Autodesk Inventor part; units mm, degrees
ref_plane "YZ Plane" through (0, 0, 0) normal (1, 0, 0) x (0, 1, 0)
ref_plane "XZ Plane" through (0, 0, 0) normal (0, 1, 0) x (-1, 0, 0)
ref_plane "XY Plane" through (0, 0, 0) normal (0, 0, 1) x (1, 0, 0)
sketch "Sketch1" plane through (0, 0, 0) normal (0, 0, 1) x (1, 0, 0)
  line L0 (-150, -75) -> (150, -75) construction
  line L1 (150, -75) -> (150, 75) construction
  line L2 (150, 75) -> (-150, 75) construction
  line L3 (-150, 75) -> (-150, -75) construction
  line L4 (-150, -75) -> (150, 75) construction
  line L5 (150, -75) -> (-150, 75) construction
  line L6 (147.5, -72.5) -> (-147.5, -72.5) construction
  line L7 (-147.5, -72.5) -> (-147.5, 72.5) construction
  line L8 (-147.5, 72.5) -> (147.5, 72.5) construction
  line L9 (147.5, 72.5) -> (147.5, -72.5) construction
  line L10 (147.5, -72.5) -> (-147.5, 72.5) construction
  line L11 (-147.5, -72.5) -> (147.5, 72.5) construction
  line L12 (-150, 75) -> (-146, 75) construction
  line L13 (-146, 75) -> (-146, 71) construction
  line L14 (-146, 71) -> (-150, 71) construction
  line L15 (-150, 71) -> (-150, 75) construction
  arc A0 (-146, 75) -> (-150, 71) centre (-146, 71) ccw
  line L16 (-150, -75) -> (-146, -75) construction
  line L17 (-146, -75) -> (-146, -71) construction
  line L18 (-146, -71) -> (-150, -71) construction
  line L19 (-150, -71) -> (-150, -75) construction
  line L20 (150, -75) -> (146, -75) construction
  line L21 (146, -75) -> (146, -71) construction
  line L22 (146, -71) -> (150, -71) construction
  line L23 (150, -71) -> (150, -75) construction
  line L24 (150, 75) -> (146, 75) construction
  line L25 (146, 75) -> (146, 71) construction
  line L26 (146, 71) -> (150, 71) construction
  line L27 (150, 71) -> (150, 75) construction
  line L28 (-146, 75) -> (146, 75)
  arc A1 (150, 71) -> (146, 75) centre (146, 71) ccw
  line L29 (150, 71) -> (150, -71)
  arc A2 (146, -75) -> (150, -71) centre (146, -71) ccw
  line L30 (146, -75) -> (-146, -75)
  arc A3 (-150, -71) -> (-146, -75) centre (-146, -71) ccw
  line L31 (-150, -71) -> (-150, 71)
  circle A4 centre (-146, 71) radius 2.5
  circle A5 centre (-146, -71) radius 2.5
  circle A6 centre (146, -71) radius 2.5
  circle A7 centre (146, 71) radius 2.5
  line L32 (-146, 71) -> (-142, 71) construction
  line L33 (-142, 71) -> (-142, 67) construction
  line L34 (-142, 67) -> (-146, 67) construction
  line L35 (-146, 67) -> (-146, 71) construction
  line L36 (-146, -71) -> (-142, -71) construction
  line L37 (-142, -71) -> (-142, -67) construction
  line L38 (-142, -67) -> (-146, -67) construction
  line L39 (-146, -67) -> (-146, -71) construction
  line L40 (146, -71) -> (142, -71) construction
  line L41 (142, -71) -> (142, -67) construction
  line L42 (142, -67) -> (146, -67) construction
  line L43 (146, -67) -> (146, -71) construction
  line L44 (146, 71) -> (142, 71) construction
  line L45 (142, 71) -> (142, 67) construction
  line L46 (142, 67) -> (146, 67) construction
  line L47 (146, 67) -> (146, 71) construction
  arc A8 (-146, 67) -> (-142, 71) centre (-146, 71) ccw
  arc A9 (-142, -71) -> (-146, -67) centre (-146, -71) ccw
  arc A10 (146, -67) -> (142, -71) centre (146, -71) ccw
  arc A11 (142, 71) -> (146, 67) centre (146, 71) ccw
  line L48 (-142, 71) -> (-140.5, 71) construction
  line L49 (-140.5, 71) -> (-140.5, 72.5) construction
  line L50 (-140.5, 72.5) -> (-142, 72.5) construction
  line L51 (-142, 72.5) -> (-142, 71) construction
  line L52 (-146, 67) -> (-147.5, 67) construction
  line L53 (-147.5, 67) -> (-147.5, 65.5) construction
  line L54 (-147.5, 65.5) -> (-146, 65.5) construction
  line L55 (-146, 65.5) -> (-146, 67) construction
  line L56 (142, 71) -> (140.5, 71) construction
  line L57 (140.5, 71) -> (140.5, 72.5) construction
  line L58 (140.5, 72.5) -> (142, 72.5) construction
  line L59 (142, 72.5) -> (142, 71) construction
  line L60 (146, 67) -> (147.5, 67) construction
  line L61 (147.5, 67) -> (147.5, 65.5) construction
  line L62 (147.5, 65.5) -> (146, 65.5) construction
  line L63 (146, 65.5) -> (146, 67) construction
  line L64 (146, -67) -> (147.5, -67) construction
  line L65 (147.5, -67) -> (147.5, -65.5) construction
  line L66 (147.5, -65.5) -> (146, -65.5) construction
  line L67 (146, -65.5) -> (146, -67) construction
  line L68 (142, -71) -> (140.5, -71) construction
  line L69 (140.5, -71) -> (140.5, -72.5) construction
  line L70 (140.5, -72.5) -> (142, -72.5) construction
  line L71 (142, -72.5) -> (142, -71) construction
  line L72 (-142, -71) -> (-140.5, -71) construction
  line L73 (-140.5, -71) -> (-140.5, -72.5) construction
  line L74 (-140.5, -72.5) -> (-142, -72.5) construction
  line L75 (-142, -72.5) -> (-142, -71) construction
  line L76 (-146, -67) -> (-147.5, -67) construction
  line L77 (-147.5, -67) -> (-147.5, -65.5) construction
  line L78 (-147.5, -65.5) -> (-146, -65.5) construction
  line L79 (-146, -65.5) -> (-146, -67) construction
  arc A12 (-147.5, -65.5) -> (-146, -67) centre (-146, -65.5) ccw
  arc A13 (-142, -71) -> (-140.5, -72.5) centre (-140.5, -71) ccw
  arc A14 (-140.5, 72.5) -> (-142, 71) centre (-140.5, 71) ccw
  arc A15 (-146, 67) -> (-147.5, 65.5) centre (-146, 65.5) ccw
  arc A16 (140.5, -72.5) -> (142, -71) centre (140.5, -71) ccw
  arc A17 (146, -67) -> (147.5, -65.5) centre (146, -65.5) ccw
  line L80 (147.5, -65.5) -> (147.5, 65.5)
  arc A18 (147.5, 65.5) -> (146, 67) centre (146, 65.5) ccw
  arc A19 (142, 71) -> (140.5, 72.5) centre (140.5, 71) ccw
  line L81 (140.5, 72.5) -> (-140.5, 72.5)
  line L82 (-147.5, 65.5) -> (-147.5, -65.5)
  line L83 (-140.5, -72.5) -> (140.5, -72.5)
  line L84 (146, 75) -> (-146, 75)
  arc A20 (-146, 75) -> (-150, 71) centre (-146, 71) ccw
  line L85 (-150, 71) -> (-150, -71)
  arc A21 (-150, -71) -> (-146, -75) centre (-146, -71) ccw
  line L86 (-146, -75) -> (146, -75)
  arc A22 (146, -75) -> (150, -71) centre (146, -71) ccw
  line L87 (150, -71) -> (150, 71)
  arc A23 (150, 71) -> (146, 75) centre (146, 71) ccw
  arc A24 (142, 71) -> (146, 67) centre (146, 71) ccw
  arc A25 (142, 71) -> (140.5, 72.5) centre (140.5, 71) ccw
  line L88 (140.5, 72.5) -> (-140.5, 72.5)
  arc A26 (-140.5, 72.5) -> (-142, 71) centre (-140.5, 71) ccw
  arc A27 (-146, 67) -> (-142, 71) centre (-146, 71) ccw
  arc A28 (-146, 67) -> (-147.5, 65.5) centre (-146, 65.5) ccw
  line L89 (-147.5, 65.5) -> (-147.5, -65.5)
  arc A29 (-147.5, -65.5) -> (-146, -67) centre (-146, -65.5) ccw
  arc A30 (-142, -71) -> (-146, -67) centre (-146, -71) ccw
  arc A31 (-142, -71) -> (-140.5, -72.5) centre (-140.5, -71) ccw
  line L90 (-140.5, -72.5) -> (140.5, -72.5)
  arc A32 (140.5, -72.5) -> (142, -71) centre (140.5, -71) ccw
  arc A33 (146, -67) -> (142, -71) centre (146, -71) ccw
  arc A34 (146, -67) -> (147.5, -65.5) centre (146, -65.5) ccw
  line L91 (147.5, -65.5) -> (147.5, 65.5)
  arc A35 (147.5, 65.5) -> (146, 67) centre (146, 65.5) ccw
  line L92 (-147.5, 72.5) -> (-140.5, 72.5) construction
  line L93 (-140.5, 72.5) -> (-140.5, 65.5) construction
  line L94 (-140.5, 65.5) -> (-147.5, 65.5) construction
  line L95 (-147.5, 65.5) -> (-147.5, 72.5) construction
  line L96 (-147.5, -72.5) -> (-140.5, -72.5) construction
  line L97 (-140.5, -72.5) -> (-140.5, -65.5) construction
  line L98 (-140.5, -65.5) -> (-147.5, -65.5) construction
  line L99 (-147.5, -65.5) -> (-147.5, -72.5) construction
  line L100 (147.5, -72.5) -> (140.5, -72.5) construction
  line L101 (140.5, -72.5) -> (140.5, -65.5) construction
  line L102 (140.5, -65.5) -> (147.5, -65.5) construction
  line L103 (147.5, -65.5) -> (147.5, -72.5) construction
  line L104 (140.5, 65.5) -> (147.5, 65.5) construction
  line L105 (147.5, 65.5) -> (147.5, 72.5) construction
  line L106 (147.5, 72.5) -> (140.5, 72.5) construction
  line L107 (140.5, 72.5) -> (140.5, 65.5) construction
  circle A36 centre (146, 71) radius 5.5 construction
  circle A37 centre (146, -71) radius 5.5 construction
  circle A38 centre (-146, -71) radius 5.5 construction
  circle A39 centre (-146, 71) radius 5.5 construction
  arc A40 (-146, 65.5) -> (-140.5, 71) centre (-146, 71) ccw
  arc A41 (140.5, 71) -> (146, 65.5) centre (146, 71) ccw
  line L108 (140.5, 71) -> (-140.5, 71)
  line L109 (-146, 65.5) -> (-146, -65.5)
  arc A42 (-140.5, -71) -> (-146, -65.5) centre (-146, -71) ccw
  line L110 (-140.5, -71) -> (140.5, -71)
  arc A43 (146, -65.5) -> (140.5, -71) centre (146, -71) ccw
  line L111 (146, -65.5) -> (146, 65.5)
  point P0 (0, 0)
  point P1 (0, 0)
  dimension "d0" = 300
  dimension "d1" = 150
  dimension "d2" = 295
  dimension "d3" = 145
  dimension "d4" = 4
  dimension "d5" = 4
  dimension "d6" = 4
  dimension "d7" = 4
  dimension "d8" = 4
  dimension "d9" = 4
  dimension "d10" = 4
  dimension "d11" = 4
  dimension "d12" = 4
  dimension "d13" = 4
  dimension "d14" = 4
  dimension "d15" = 4
  dimension "d16" = 5
  dimension "d17" = 5
  dimension "d18" = 5
  dimension "d19" = 5
  dimension "d20" = 4
  dimension "d21" = 4
  dimension "d22" = 4
  dimension "d23" = 4
  dimension "d24" = 4
  dimension "d25" = 4
  dimension "d26" = 4
  dimension "d27" = 4
  dimension "d28" = 4
  dimension "d29" = 4
  dimension "d30" = 4
  dimension "d31" = 4
  dimension "d32" = 1.5
  dimension "d33" = 1.5
  dimension "d34" = 1.5
  dimension "d35" = 1.5
  dimension "d36" = 1.5
  dimension "d37" = 1.5
  dimension "d38" = 1.5
  dimension "d39" = 1.5
  dimension "d40" = 1.5
  dimension "d41" = 1.5
  dimension "d42" = 1.5
  dimension "d43" = 1.5
  dimension "d44" = 1.5
  dimension "d45" = 1.5
  dimension "d46" = 1.5
  dimension "d47" = 1.5
  dimension "d48" = 1.5
  dimension "d49" = 1.5
  dimension "d50" = 1.5
  dimension "d51" = 1.5
  dimension "d52" = 1.5
  dimension "d53" = 1.5
  dimension "d54" = 1.5
  dimension "d55" = 1.5
  dimension "d60" = 9.5
  dimension "d61" = 9.5
  dimension "d62" = 140.5
  dimension "d63" = 290.5
extrude "Extrusion1" add sketch "Sketch1" along normal blind 2.5 contours L28 A1 L29 A2 L30 A3 L31 A0 | A8 A14 L81 A19 A11 A18 L80 A17 A10 A16 L83 A13 A9 A12 L82 A15 | A40 L108 A41 L111 A43 L110 A42 L109
extrude "Extrusion2" add sketch "Sketch1" along normal blind 0.5 contours A4 | A5 | A6 | A7
extrude "Extrusion3" add sketch "Sketch1" along normal blind 5 contours A8 A14 L81 A19 A11 A18 L80 A17 A10 A16 L83 A13 A9 A12 L82 A15
equation "\"d21\" = d20"
properties part number "electronics_box_cap"
Build history of the part. All positions in model axes, mm. Round coordinates to 2 decimals unless told otherwise and drop trailing zeros. Order: outer loops, then holes, each group sorted by start corner. A loop starts at its lowest first (then second) coordinate and runs counter-clockwise, first axis right, second up. Notation, with made-up numbers: (84.5, 73.25) -> (110.5, 73.25) arc R30 cw to (110.5, 106.25) -> close; hole circle Ø3 at (89.5, 36). An arc over 180 degrees is marked (long way). Answer in a Markdown table with one row per item.
1) Band-saw the part on A-A on z = 3.4. Give the cut face in (x, y).
Values:
| item | result |
|---|---|
| outline | (-147.5, -65.5) arc R1.5 ccw to (-146, -67) arc R4 cw to (-142, -71) arc R1.5 ccw to (-140.5, -72.5) -> (140.5, -72.5) arc R1.5 ccw to (142, -71) arc R4 cw to (146, -67) arc R1.5 ccw to (147.5, -65.5) -> (147.5, 65.5) arc R1.5 ccw to (146, 67) arc R4 cw to (142, 71) arc R1.5 ccw to (140.5, 72.5) -> (-140.5, 72.5) arc R1.5 ccw to (-142, 71) arc R4 cw to (-146, 67) arc R1.5 ccw to (-147.5, 65.5) -> close; hole (-146, -65.5) arc R5.5 cw to (-140.5, -71) -> (140.5, -71) arc R5.5 cw to (146, -65.5) -> (146, 65.5) arc R5.5 cw to (140.5, 71) -> (-140.5, 71) arc R5.5 cw to (-146, 65.5) -> close |
2) Band-saw the part on B-B on y = -2. Give the cut face in (x, z).
Values:
| item | result |
|---|---|
| outline | (-150, 0) -> (150, 0) -> (150, 2.5) -> (147.5, 2.5) -> (147.5, 5) -> (146, 5) -> (146, 2.5) -> (-146, 2.5) -> (-146, 5) -> (-147.5, 5) -> (-147.5, 2.5) -> (-150, 2.5) -> close |
3) Wall check: L1, parallel to Y at x = 146, z = 1.4; L2, parallel to Y at x = 49.5, z = 4.55; L3, parallel to X at y = 52.5, z = 4.5. Give the ranges that are in metal, low to high.
Values:
| item | result |
|---|---|
| L1 | -75 to -73.5, -68.5 to 68.5, 73.5 to 75 |
| L2 | -72.5 to -71, 71 to 72.5 |
| L3 | -147.5 to -146, 146 to 147.5 |
4) Mould opens along Y. For faces 1 (the flat face through (-2, 1, 0)), 2 (the cylindrical face through (-142.07, 67.15, 3.73)), 3 (the cylindrical face through (142.15, 67.07, 3.73)) say: released by +Y, released by -Y, zero draft, split by the parting line, or undercut.
Values:
| item | result |
|---|---|
| face 1 | zero draft |
| face 2 | undercut |
| face 3 | undercut |
5) Pin check, flat tips, straight feed: P1, Ø1.5, axis at x = -145.5, y = 71, coming from the +Z side; P2, Ø1.2, axis at y = 17, z = 4.5, coming from the -X side; P3, Ø2, axis at x = 64.5, z = 4, coming from the +Y side. Stop position of each tip, or through.
Values:
| item | result |
|---|---|
| P1 | z = 0.5 |
| P2 | x = -147.5 |
| P3 | y = 72.5 |
6) Band-saw the part on C-C on x = 70. Give the cut face in (y, z).
Values:
| item | result |
|---|---|
| outline | (-75, 0) -> (75, 0) -> (75, 2.5) -> (72.5, 2.5) -> (72.5, 5) -> (71, 5) -> (71, 2.5) -> (-71, 2.5) -> (-71, 5) -> (-72.5, 5) -> (-72.5, 2.5) -> (-75, 2.5) -> close |
